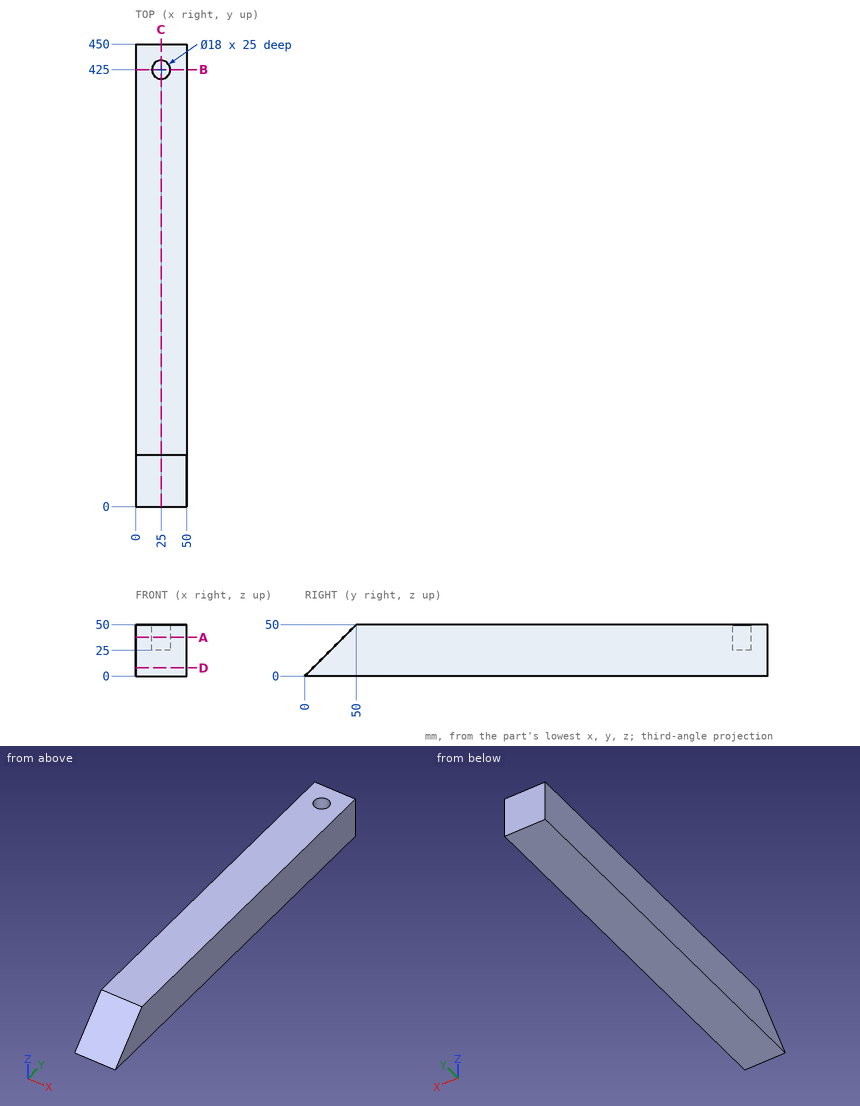
Answer from the drawing. Dimensions are ordinates in mm from the lowest x, y and z of the part. Give positions to 0.01 mm unless a question says otherwise; leave off trailing zeros. Write each loop counter-clockwise with the first axis right and the second up, starting at its lowest first coordinate (ties: lowest second). Pieces come first, ordered by that corner, then holes.
1) Find the intervals of material crossed by L1, parallel to Y at x = 25, z = 31; L2, parallel to Y at x = 25, z = 32.75; L3, parallel to Y at x = 46.5, z = 29.5, in increasing order.
2) Section B-B (y = 425) is taken. Write down the section's boundary in (x, z), and give its area (3 significant figures).
3) Section D-D (z = 8) is taken. Write down the section's boundary in (x, y).
4) Section C-C (x = 25) is taken. Write down the section's boundary in (y, z).
5) Section A-A (z = 37.5) is taken. Write down the section's boundary in (x, y).
6) Given P1, Ø2, axis at x = 34.5, z = 42.5, coming from the -Y side; P2, Ø9, axis at x = 22.5, y = 424, coming from the +Z side, each flat-ended and moving along its own axis, determine where each tip first touches the part or whether it passes through.
Response:
1. L1: y = 31 to 416, 434 to 450
1. L2: y = 32.75 to 416, 434 to 450
1. L3: y = 29.5 to 450
2. outline: (0, 0) - (50, 0) - (50, 50) - (34, 50) - (34, 25) - (16, 25) - (16, 50) - (0, 50) - close
2. area: 2,050 mm2
3. outline: (0, 8) - (50, 8) - (50, 450) - (0, 450) - close
4. outline: (0, 0) - (450, 0) - (450, 50) - (434, 50) - (434, 25) - (416, 25) - (416, 50) - (50, 50) - close
5. outline: (0, 37.5) - (50, 37.5) - (50, 450) - (0, 450) - close; hole circle Ø18 at (25, 425)
6. P1: stops at y = 41.5
6. P2: stops at z = 25
